```python
from build123d import *

# Parameters (mm, degrees)
SKETCH1_R                      = 2.25
SKETCH1_R_2                    = 8.125
BOSS_EXTRUDE1_DEPTH            = 44
CUT_EXTRUDE1_DEPTH             = 4
CUT_EXTRUDE3_DEPTH             = 84.822822817
CUT_EXTRUDE3_DEPTH_BACK        = 84.822822817
F_4_5_4_5_DIAMETER_HOLE1_D     = 4.5
F_4_5_4_5_DIAMETER_HOLE1_DEPTH = 10
F_4_5_4_5_DIAMETER_HOLE1_TIP   = 1.351936393
F_3_3_3_3_DIAMETER_HOLE1_D     = 3.3
CUT_EXTRUDE4_DEPTH             = 84.822822817
CUT_EXTRUDE4_DEPTH_BACK        = 84.822822817
CHAMFER1_SIZE                  = 1


with BuildPart() as part:
    # Sketch1 → Boss-Extrude1 (new body)
    with BuildSketch(Plane(origin=(0, 0, 0), x_dir=(1, 0, 0), z_dir=(0, 1, 0))):
        with BuildLine():
            Line((-7.323571846, 63.6171875), (-15.74567947, 25.476953125))
            ThreePointArc((-15.74567947, 25.476953125), (-16.107587682, 22.749162244), (-16.000432679, 19.99955528))
            Line((-16.000432679, 19.99955528), (-13.5, 0))
            Line((-13.5, 0), (13.5, 0))
            Line((13.5, 0), (16.000432679, 19.99955528))
            ThreePointArc((16.000432679, 19.99955528), (16.107587682, 22.749162244), (15.74567947, 25.476953125))
            Line((15.74567947, 25.476953125), (7.323571846, 63.6171875))
            ThreePointArc((7.323571846, 63.6171875), (0, 69.5), (-7.323571846, 63.6171875))
        make_face()
        with Locations(Location((0, 62, 0), (0, 0, 270))):
            Circle(SKETCH1_R, mode=Mode.SUBTRACT)
        with Locations(Location((0, 22, 0), (0, 0, 270))):
            Circle(SKETCH1_R_2, mode=Mode.SUBTRACT)
    extrude(amount=BOSS_EXTRUDE1_DEPTH)

    # Sketch2 → Cut-Extrude1 (cut)
    with BuildSketch(Plane.XZ):
        with BuildLine():
            Line((-15.74567947, -25.476953125), (-12.952744037, -38.125))
            Line((-12.952744037, -38.125), (12.952744037, -38.125))
            Line((12.952744037, -38.125), (15.74567947, -25.476953125))
            ThreePointArc((15.74567947, -25.476953125), (16.107587682, -22.749162244), (16.000432679, -19.99955528))
            Line((16.000432679, -19.99955528), (13.5, 0))
            Line((13.5, 0), (-13.5, 0))
            Line((-13.5, 0), (-16.000432679, -19.99955528))
            ThreePointArc((-16.000432679, -19.99955528), (-16.107587682, -22.749162244), (-15.74567947, -25.476953125))
        make_face()
    extrude(amount=-CUT_EXTRUDE1_DEPTH, mode=Mode.SUBTRACT)

    # Sketch3 → Cut-Extrude3 (cut, two sides: drawn at the far end of the back side and taken through both)
    with BuildSketch(Plane(origin=(0, 0, 0), x_dir=(0, 0, -1), z_dir=(1, 0, 0)).offset(-CUT_EXTRUDE3_DEPTH_BACK)):
        Polygon((69.5, 37), (69.5, 0), (38.125, 0), (38.125, 4), align=None)
    extrude(amount=CUT_EXTRUDE3_DEPTH + CUT_EXTRUDE3_DEPTH_BACK, mode=Mode.SUBTRACT)

    # Ø4.5 (4.5) Diameter Hole1
    with Locations(Plane(origin=(0, 4, 0), x_dir=(-1, 0, 0), z_dir=(0, -1, 0))):
        with Locations((12, 22), (0, 34), (-12, 22), (0, 10)):
            Hole(F_4_5_4_5_DIAMETER_HOLE1_D / 2, depth=F_4_5_4_5_DIAMETER_HOLE1_DEPTH)
            with Locations((0, 0, -(F_4_5_4_5_DIAMETER_HOLE1_DEPTH + F_4_5_4_5_DIAMETER_HOLE1_TIP / 2))):  # 118° drill point
                Cone(0, F_4_5_4_5_DIAMETER_HOLE1_D / 2, F_4_5_4_5_DIAMETER_HOLE1_TIP, mode=Mode.SUBTRACT)

    # Ø3.3 (3.3) Diameter Hole1 (through all)
    with Locations(Plane.XY):
        with Locations((-10, 32), (10, 32), (10, 12), (-10, 12)):
            Hole(F_3_3_3_3_DIAMETER_HOLE1_D / 2)

    # Sketch10 → Cut-Extrude4 (cut, two sides: drawn at the far end of the back side and taken through both)
    with BuildSketch(Plane(origin=(0, 0, 0), x_dir=(0, 0, -1), z_dir=(1, 0, 0)).offset(-CUT_EXTRUDE4_DEPTH_BACK)):
        with BuildLine():
            Line((10, 35.5), (25, 35.5))
            ThreePointArc((25, 35.5), (28.5, 32), (25, 28.5))
            Line((25, 28.5), (10, 28.5))
            Line((10, 28.5), (10, 35.5))
        make_face()
        with BuildLine():
            Line((10, 15.5), (25, 15.5))
            ThreePointArc((25, 15.5), (28.5, 12), (25, 8.5))
            Line((25, 8.5), (10, 8.5))
            Line((10, 8.5), (10, 15.5))
        make_face()
    extrude(amount=CUT_EXTRUDE4_DEPTH + CUT_EXTRUDE4_DEPTH_BACK, mode=Mode.SUBTRACT)

    # Chamfer1
    chamfer1_edges = [part.edges().sort_by_distance(p)[0] for p in [
        (-14.25, 4, -22),
        (0, 44, -64.25),
        (-2.25, 4, -10),
        (9.75, 4, -22),
        (-2.25, 4, -34),
    ]]
    chamfer(chamfer1_edges, length=CHAMFER1_SIZE)


solid = part.part
```
For this review, take the finished solid that the model builds, in its own axes (mm). A direction names the side the tool comes from. Round coordinates to 2 decimals unless told otherwise and drop trailing zeros. Order: outer loops, then holes, each group sorted by start corner. A loop starts at its lowest first (then second) coordinate and runs counter-clockwise, first axis right, second up. Notation, with made-up numbers: (70.5, 84.5) -> (123.5, 84.5) arc R18 cw to (123.5, 116.5) -> close; hole circle Ø3 at (36.25, 39.25). An arc over 180 degrees is marked (long way). Use a Markdown table: item, result.
Item 1: For pin 1 (1.5 mm diameter, centred on y = 22.5, z = -56.5, fed in from -X); pin 2 (4 mm diameter, centred on x = -12, z = -22, fed in from -Y); pin 3 (7.5 mm diameter, centred on x = 2, y = 33.5, fed in from -Z); pin 4 (2 mm diameter, centred on x = 10, y = 12, fed in from -Z), all flat-tipped, find the tip position at first contact; note any pin that passes through.
Resolved:
| item | result |
|---|---|
| pin 1 | stops at x = -9.06 |
| pin 2 | stops at y = 15.5 |
| pin 3 | stops at z = -69.48 |
| pin 4 | passes through |
Item 2: Take a section at A-A (y = 12). State the section outline as (x, z) points (3 decimals), plus the area to 3 significant figures.
Resolved:
| item | result |
|---|---|
| outline | (-15.078, -28.5) -> (-11.65, -44.025) -> (-11.65, -28.5) -> close; (-14.75, -10) -> (-11.65, -10) -> (-11.65, 0) -> (-13.5, 0) -> close; (-8.35, -45.731) -> (8.35, -45.731) -> (8.35, -28.5) -> (4.875, -28.5) arc R8.125 cw to (-4.875, -28.5) -> (-8.35, -28.5) -> close; (-8.35, -10) -> (-2.25, -10) arc R2.25 cw to (2.25, -10) -> (8.35, -10) -> (8.35, 0) -> (-8.35, 0) -> close; (11.65, -44.025) -> (15.078, -28.5) -> (11.65, -28.5) -> close; (11.65, -10) -> (14.75, -10) -> (13.5, 0) -> (11.65, 0) -> close; hole circle Ø4.5 at (0, -34) |
| area | 523 mm² |
Item 3: Machinability: for faces 5 (the cylindrical face through (-12.488, 6.774, -19.804)), 6 (the cylindrical face through (16.11, 6.23, -22.71)), 7 (the cylindrical face through (11.501, 30.876, -28.314)), which of the approach directions +Z, -Z, +X, -X, +Y, -Y give a long, thin tool a straight path to every point of the face, cutting with its end or side? Answer none if there is none.
Resolved:
| item | result |
|---|---|
| face 5 | -Y |
| face 6 | +X, +Y, -Y |
| face 7 | +X, -X |
Item 4: Draft analysis for pull direction Y (two halves, no side actions). For faces 1 (the cylindrical face through (-11.65, 33.27, -28.26)), 2 (the flat face through (0, 32, -10)), 3 (the flat face through (0, 44, -35)), 4 (the cylindrical face through (1.038, 8.563, -8.004)), state which applies: +Y half, -Y half, draft (parallel to the pull), parting line (faces both ways), or undercut.
Resolved:
| item | result |
|---|---|
| face 1 | undercut |
| face 2 | undercut |
| face 3 | +Y half |
| face 4 | draft |
Item 5: For line 1 along Y through (x, z) = (6, -14.5); line 2 along Z through (x, y) = (0, 37.5) (3 decimals); line 3 along Y through (x, z) = (-10, -2.25), list the stretches that pass through material, from the lowest coordinate up. Write a range as [from, to].
Resolved:
| item | result |
|---|---|
| line 1 | y = [4, 8.5], [15.5, 28.5], [35.5, 44] |
| line 2 | z = [-69.5, -64.25], [-59.75, -30.125], [-13.875, 0] |
| line 3 | y = [4, 10.35], [13.65, 30.35], [33.65, 44] |
Item 6: Take a section at D-D (y = 23). State the section outline as (x, z) points (3 decimals).
Resolved:
| item | result |
|---|---|
| outline | (-16, -20) arc R16.125 ccw to (-15.746, -25.477) -> (-8.964, -56.189) -> (8.964, -56.189) -> (15.746, -25.477) arc R16.125 ccw to (16, -20) -> (13.5, 0) -> (-13.5, 0) -> close; hole circle Ø16.25 at (0, -22) |
Item 7: Take a section at B-B (z = -62). State the section outline as (x, y) points.
Resolved:
| item | result |
|---|---|
| outline | (-7.68, 29.11) -> (-2.25, 29.11) -> (-2.25, 43) -> (-3.25, 44) -> (-7.68, 44) -> close; (2.25, 29.11) -> (7.68, 29.11) -> (7.68, 44) -> (3.25, 44) -> (2.25, 43) -> close |
Item 8: Take a section at C-C (x = -6). State the section outline as (y, z) points (3 decimals), plus the area to 3 significant figures.
Resolved:
| item | result |
|---|---|
| outline | (4, -38.125) -> (33.845, -66.5) -> (44, -66.5) -> (44, -27.479) -> (34.471, -27.479) arc R3.5 cw to (29.529, -27.479) -> (14.471, -27.479) arc R3.5 cw to (9.529, -27.479) -> (4, -27.479) -> close; (4, -16.521) -> (8.5, -16.521) -> (8.5, -10) -> (15.5, -10) -> (15.5, -16.521) -> (28.5, -16.521) -> (28.5, -10) -> (35.5, -10) -> (35.5, -16.521) -> (44, -16.521) -> (44, 0) -> (4, 0) -> close |
| area | 1,700 mm² |
